from build123d import *

# Parameters (mm, degrees)
BOSS_EXTRUDE1_DEPTH = 2
SKETCH3_R           = 5
BOSS_EXTRUDE2_DEPTH = 2
SKETCH5_W           = 12
SKETCH5_H           = 10
BOSS_EXTRUDE3_DEPTH = 5


with BuildPart() as part:
    # Sketch2 → Boss-Extrude1 (new body)
    with BuildSketch(Plane(origin=(0, 0, 0), x_dir=(1, 0, 0), z_dir=(0, 1, 0))):
        with BuildLine():
            Line((2.043336986, 20), (10, 20))
            Line((10, 20), (10, -8))
            ThreePointArc((10, -8), (12, -10), (10, -12))
            Line((10, -12), (10, -20))
            Line((10, -20), (-10, -20))
            Line((-10, -20), (-10, -12))
            ThreePointArc((-10, -12), (-12, -10), (-10, -8))
            Line((-10, -8), (-10, 20))
            Line((-10, 20), (-2.043336986, 20))
            ThreePointArc((-2.043336986, 20), (0, 22.043336986), (2.043336986, 20))
        make_face()
    extrude(amount=BOSS_EXTRUDE1_DEPTH)

    # Sketch3 → Boss-Extrude2 (add)
    with BuildSketch(Plane(origin=(0, 2, 0), x_dir=(1, 0, 0), z_dir=(0, 1, 0))):
        with Locations(Location((0, 10, 0), (0, 0, 270))):
            Circle(SKETCH3_R)
    extrude(amount=BOSS_EXTRUDE2_DEPTH)

    # Sketch5 → Boss-Extrude3 (add)
    with BuildSketch(Plane.XZ):
        with Locations((0, 15)):
            Rectangle(SKETCH5_W, SKETCH5_H)
    extrude(amount=BOSS_EXTRUDE3_DEPTH)


solid = part.part
Design review of the part built by this model. Coordinates are the model's own, in mm. A direction names the side the tool comes from. Coordinates: 2 decimals unless noted, no trailing zeros. Write each loop counter-clockwise with the first axis right and the second up, starting at its lowest first coordinate (ties: lowest second). Pieces come first, ordered by that corner, then holes. Notation, with made-up numbers: (-4.75, 70.5) - (5.25, 70.5) arc R18 ccw to (5.25, 76.5) - close; hole circle Ø3 at (64, 89). An arc over 180 degrees is marked (long way). One line per item, written item: value.
1) Add section A-A (x = 0). State the section outline as (y, z) points.
Answer sheet:
outline: (-5, 10) - (0, 10) - (0, -22.04) - (2, -22.04) - (2, -15) - (4, -15) - (4, -5) - (2, -5) - (2, 20) - (-5, 20) - close
2) Add section B-B (y = 1.25). State the section outline as (x, z) points.
Answer sheet:
outline: (-10, -20) - (-2.04, -20) arc R2.04 ccw to (2.04, -20) - (10, -20) - (10, 8) arc R2 ccw to (10, 12) - (10, 20) - (-10, 20) - (-10, 12) arc R2 ccw to (-10, 8) - close
3) Add section D-D (z = -10). State the section outline as (x, y) points, plus the area to 3 significant figures.
Answer sheet:
outline: (-10, 0) - (10, 0) - (10, 2) - (5, 2) - (5, 4) - (-5, 4) - (-5, 2) - (-10, 2) - close
area: 60.0 mm2
4) Add section C-C (z = 17). State the section outline as (x, y) points.
Answer sheet:
outline: (-10, 0) - (-6, 0) - (-6, -5) - (6, -5) - (6, 0) - (10, 0) - (10, 2) - (-10, 2) - close
5) To check wall thickness, follow probe 1 along X at (y, z) = (1.25, 0.5); probe 2 along Y at (x, z) = (5.5, 12); probe 3 along Z at (x, y) = (8, 1.75). State the ranges of each line that lie inside material, in increasing order.
Answer sheet:
probe 1: x = -10 to 10
probe 2: y = -5 to 2
probe 3: z = -20 to 20
6) Insertion check: pin 1 (1 mm diameter, centred on x = 6, z = -15, fed in from +Y); pin 2 (2.5 mm diameter, centred on x = -2, y = -1.5, fed in from -Z); pin 3 (1 mm diameter, centred on y = 1, z = -7.5, fed in from +X). Each pin has a flat end and moves straight along its axis. Give the tip position at first contact, or say it passes through.
Answer sheet:
pin 1: stops at y = 2
pin 2: stops at z = 10
pin 3: stops at x = 10
7) For faces 1 (the face through (-10, 1, 16)), 2 (the face through (0, -2, 10)), 3 (the face through (-6, -2, 15)), 4 (the face through (-6, 1, -20)), list the 3-axis set-ups (+Z, -Z, +X, -X, +Y, -Y) from which the entire face can be reached by the end or side of a thin tool; tool diameter is ignored.
Answer sheet:
face 1: +Z, -X, +Y, -Y
face 2: -Z, +X, -X, -Y
face 3: +Z, -Z, -X, -Y
face 4: -Z, -X, +Y, -Y
